Source: CAD feature listing. Evaluate the final solid. Frame: model axes, mm. Round coordinates to 2 decimals unless told otherwise and drop trailing zeros. Write each loop counter-clockwise with the first axis right and the second up, starting at its lowest first coordinate (ties: lowest second). Pieces come first, ordered by that corner, then holes. Notation, with made-up numbers: (-18, 13) -> (30, 13) arc R16 ccw to (30, 25) -> close; hole circle Ø11 at (76.25, -36). An arc over 180 degrees is marked (long way). Return JSON: item names as keys, results as strings. Group by question number.
from build123d import *

# Parameters (mm, degrees)
ESQUISSE1_R        = 1.5
BOSS_EXTRU_1_DEPTH = 10


with BuildPart() as part:
    # Esquisse1 → Boss.-Extru.1 (new body)
    with BuildSketch(Plane(origin=(0, 0, 0), x_dir=(1, 0, 0), z_dir=(0, 1, 0))):
        Polygon((2.886751346, 0), (1.443375673, 2.5), (-1.443375673, 2.5), (-2.886751346, 0), (-1.443375673, -2.5), (1.443375673, -2.5), align=None)
        with Locations(Location((0, 0, 0), (0, 0, 270))):
            Circle(ESQUISSE1_R, mode=Mode.SUBTRACT)
    extrude(amount=BOSS_EXTRU_1_DEPTH)

    # Esquisse3 → Enlèvement de matière-Révolution1 (revolve, cut)
    with BuildSketch(Plane.XY, mode=Mode.PRIVATE) as enl_vement_de_mati_re_r_volution1_sk:
        with BuildLine():
            Line((2.386751346, 10), (2.886751346, 10))
            Line((2.886751346, 10), (2.886751346, 9.5))
            ThreePointArc((2.886751346, 9.5), (2.740304737, 9.853553391), (2.386751346, 10))
        make_face()
        with BuildLine():
            Line((2.886751346, 0.5), (2.886751346, 0))
            Line((2.886751346, 0), (2.386751346, 0))
            ThreePointArc((2.386751346, 0), (2.740304737, 0.146446609), (2.886751346, 0.5))
        make_face()
    revolve(enl_vement_de_mati_re_r_volution1_sk.sketch.rotate(Axis((0, -0.5, 0), (0, 1, 0)), 90), axis=Axis((0, -0.5, 0), (0, 1, 0)), mode=Mode.SUBTRACT)


solid = part.part
Item 1: First-contact query: pin 1 Ø1 at (x, z) = (1.5, 1.5) entering from -Y; pin 2 Ø2.5 at (x, z) = (0, 0) entering from +Y. Flat tips, straight axial feed; report the tip coordinate or a pass-through.
Item 2: Cut plane C-C on y = 9.75. Output: boundary loops of the cut face in (x, z).
Item 3: Material intervals for probe 1 along Z at (x, y) = (0.4, 1); probe 2 along X at (y, z) = (4.25, 1.1); probe 3 along Z at (x, y) = (0.35, 6), sorted ascending.
Item 4: Cut plane B-B on x = 0. Output: boundary loops of the cut face in (y, z).
Item 5: Cut plane A-A on y = 1. Output: boundary loops of the cut face in (x, z).
Item 6: Pull-direction query (Z, two-part tool) for faces 1 (the flat face through (0, 0, 2)), 2 (the cylindrical face through (0.45, 4.93, 1.43)), 3 (the flat face through (0, 5, -2.5)), 4 (the flat face through (2.155, 4.93, 1.268)); classes: +Z half, -Z half, draft (parallel to the pull), parting line (faces both ways), or undercut.
Here are the results:
{
 "1": {"pin 1": "stops at y = 0", "pin 2": "passes through"},
 "2": {"outline": "(-2.82, -0.12) -> (-1.51, -2.38) arc R2.82 ccw to (-1.3, -2.5) -> (1.3, -2.5) arc R2.82 ccw to (1.51, -2.38) -> (2.82, -0.12) arc R2.82 ccw to (2.82, 0.12) -> (1.51, 2.38) arc R2.82 ccw to (1.3, 2.5) -> (-1.3, 2.5) arc R2.82 ccw to (-1.51, 2.38) -> (-2.82, 0.12) arc R2.82 ccw to start; hole circle Ø3 at (0, 0)"},
 "3": {"probe 1": "z = -2.5 to -1.45, 1.45 to 2.5", "probe 2": "x = -2.25 to -1.02, 1.02 to 2.25", "probe 3": "z = -2.5 to -1.46, 1.46 to 2.5"},
 "4": {"outline": "(0, -2.39) arc R0.5 ccw to (0.01, -2.5) -> (9.99, -2.5) arc R0.5 ccw to (10, -2.39) -> (10, -1.5) -> (0, -1.5) -> close; (0, 1.5) -> (10, 1.5) -> (10, 2.39) arc R0.5 ccw to (9.99, 2.5) -> (0.01, 2.5) arc R0.5 ccw to (0, 2.39) -> close"},
 "5": {"outline": "(-2.89, 0) -> (-1.44, -2.5) -> (1.44, -2.5) -> (2.89, 0) -> (1.44, 2.5) -> (-1.44, 2.5) -> close; hole circle Ø3 at (0, 0)"},
 "6": {"face 1": "draft", "face 2": "undercut", "face 3": "-Z half", "face 4": "+Z half"}
}
